Build history of the part. All positions in model axes, mm. Face numbers are marked on the shaded views. A direction names the side the tool comes from. Coordinates: 2 decimals unless noted, no trailing zeros. Write each loop counter-clockwise with the first axis right and the second up, starting at its lowest first coordinate (ties: lowest second). Pieces come first, ordered by that corner, then holes.
```python
from build123d import *

# Parameters (mm, degrees)
SKETCH1_R                                        = 76.2
BOSS_EXTRUDE1_DEPTH                              = 25.4
CBORE_FOR_1_2_SOCKET_HEAD_CAP_SCREW1_D           = 13.49248
CBORE_FOR_1_2_SOCKET_HEAD_CAP_SCREW1_CBORE_D     = 20.6375
CBORE_FOR_1_2_SOCKET_HEAD_CAP_SCREW1_CBORE_DEPTH = 12.7
CIRPATTERN1_COUNT                                = 8
CIRPATTERN1_ANGLE                                = 189


with BuildPart() as part:
    # Sketch1 → Boss-Extrude1 (new body)
    with BuildSketch(Plane(origin=(0, 0, 0), x_dir=(1, 0, 0), z_dir=(0, 1, 0))):
        with Locations(Location((0, 0, 0), (0, 0, 270))):
            Circle(SKETCH1_R)
    extrude(amount=BOSS_EXTRUDE1_DEPTH)

    # CBORE for 1/2 Socket Head Cap Screw1 (through all)
    with Locations(Plane(origin=(0, 25.4, 0), x_dir=(1, 0, 0), z_dir=(0, 1, 0))):
        with Locations((0, 60.325)):
            cbore_for_1_2_socket_head_cap_screw1 = CounterBoreHole(CBORE_FOR_1_2_SOCKET_HEAD_CAP_SCREW1_D / 2, CBORE_FOR_1_2_SOCKET_HEAD_CAP_SCREW1_CBORE_D / 2, CBORE_FOR_1_2_SOCKET_HEAD_CAP_SCREW1_CBORE_DEPTH)

    # CirPattern1: CBORE for 1/2 Socket Head Cap Screw1 ×8 about axis
    cirpattern1_axis = Axis((0, 0, 0), (0, -1, 0))
    for i in range(1, CIRPATTERN1_COUNT):
        add(cbore_for_1_2_socket_head_cap_screw1.rotate(cirpattern1_axis, i * CIRPATTERN1_ANGLE / (CIRPATTERN1_COUNT - 1)), mode=Mode.SUBTRACT)


solid = part.part
```
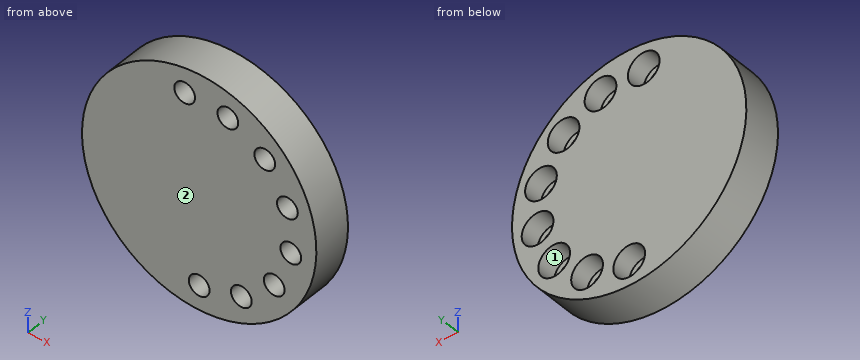
1. 3-axis set-ups, long thin cutter, end or side, ignore diameter. For the marked faces 1 and 2: which of +Z, -Z, +X, -X, +Y, -Y reach the whole face in a straight line?
Computed values:
face 1: +Y
face 2: +Z, -Z, +X, -X, -Y
2. Saw through at A-A on y = 15. State how many separate pieces and enclosed holes the cut face has, plus the area to 3 significant figures.
Computed values:
separate pieces: 1
enclosed holes: 8
area: 15,600 mm2
3. Flat gauge pins, fed straight in: pin 1 (6 mm diameter, centred on y = 5, z = -23.5, fed in from +X); pin 2 (15.5 mm diameter, centred on x = -9.44, z = 59.58, fed in from +Y); pin 3 (10 mm diameter, centred on y = 15, z = -6, fed in from +X). Where does each tip first touch, or does it go through?
Computed values:
pin 1: stops at x = 73.39
pin 2: stops at y = 12.7
pin 3: stops at x = 76.19
4. Probe line 1 along X through (y, z) = (16, -54); line 2 along Z through (x, y) = (-3.5, 8.5); line 3 along Z through (x, y) = (48, 20.5). List the from-to ranges inside material, lowest first.
Computed values:
line 1: x = -53.76 to -8.15, 8.15 to 17.07, 37.7 to 53.76
line 2: z = -76.12 to -66.09, -54.56 to 56.38, 62.79 to 76.12
line 3: z = -59.18 to -45.75, -25.17 to 14.32, 22.96 to 33.83, 51.48 to 59.18
5. Saw through at B-B on x = -27.5. List the corners of the cut face in (y, z), plus the area to 3 significant figures.
Computed values:
outline: (0, -71.06) - (25.4, -71.06) - (25.4, 71.06) - (0, 71.06) - close
area: 3,610 mm2
